from build123d import *

# Parameters (mm, degrees)
F0_W      = 711.2
F0_H      = 228.6
F0_W_2    = 685.8
F0_H_2    = 215.9
F1_DEPTH  = 381
F2_W      = 698.5
F2_H      = 136.616886
F3_DEPTH  = 190.5
F4_DEPTH  = 254
F5_W      = 203.2
F5_H      = 355.6
F6_DEPTH  = 25.4
F8_DEPTH  = 12.7
F9_W      = 698.5
F9_H      = 136.616886
F9_H_2    = 41.183114
F10_DEPTH = 381
F12_DEPTH = 25.4
F13_W     = 25.4
F13_H     = 381
F14_DEPTH = 6.35
F15_W     = 215.9
F15_H     = 120.65
F16_DEPTH = 25.4
F18_D     = 6.35
F20_D     = 12.7
F22_DEPTH = 6.35
F24_DEPTH = 6.35
F26_D     = 25.4
F28_DEPTH = 19.05
F30_D     = 12.7


with BuildPart() as f1:
    # F0 (on Top) → F1 (new body)
    with BuildSketch(Plane.XY):
        Rectangle(F0_W, F0_H)
        Rectangle(F0_W_2, F0_H_2, mode=Mode.SUBTRACT)
    extrude(amount=F1_DEPTH)

    # F2 (on face) → F3 (cut, symmetric)
    with BuildSketch(Plane.XZ.offset(114.3)):
        with Locations((0, 306.341557)):
            Rectangle(F2_W, F2_H)
    extrude(amount=F3_DEPTH, both=True, mode=Mode.SUBTRACT)

    # F2 (on face) → F4 (cut, symmetric)
    with BuildSketch(Plane.XZ.offset(114.3)):
        with BuildLine():
            Line((355.6, 0), (355.6, 190.5))
            ThreePointArc((355.6, 190.5), (153.893772, 139.874959), (0, 0))
            Line((0, 0), (355.6, 0))
        make_face()
    extrude(amount=F4_DEPTH, both=True, mode=Mode.SUBTRACT)

    # F5 (on face) → F6 (cut)
    with BuildSketch(Plane(origin=(-355.6, 0, 0), x_dir=(0, -1, 0), z_dir=(-1, 0, 0))):
        with Locations((0, 190.5)):
            Rectangle(F5_W, F5_H)
    extrude(amount=-F6_DEPTH, mode=Mode.SUBTRACT)

    # F7 (on Top) → F8 (join)
    with BuildSketch(Plane.XY):
        Polygon((-177.723765, 88.70177), (-356.087953, 88.70177), (-355.447531, -89.342214), (-177.723765, -89.342214), align=None)
    extrude(amount=F8_DEPTH)

    # F9 (on face) → F10 (cut)
    with BuildSketch(Plane.XZ.offset(114.3)):
        with Locations((0, 306.341557)):
            Rectangle(F9_W, F9_H)
        with Locations((0, 217.441557)):
            Rectangle(F9_W, F9_H_2)
    extrude(amount=-F10_DEPTH, mode=Mode.SUBTRACT)

    # F11 (on face) → F12 (cut)
    with BuildSketch(Plane.XZ.offset(114.3)):
        with BuildLine():
            Line((-177.8, 0), (0, 0))
            ThreePointArc((0, 0), (-88.9, 88.9), (-177.8, 0))
        make_face()
    extrude(amount=-F12_DEPTH, mode=Mode.SUBTRACT)

    # F13 (on face) → F14 (join)
    with BuildSketch(Plane(origin=(-355.6, 0, 0), x_dir=(0, -1, 0), z_dir=(-1, 0, 0))):
        with Locations((0, 190.5)):
            Rectangle(F13_W, F13_H)
    extrude(amount=-F14_DEPTH)

    # F15 (on face) → F16 (cut)
    with BuildSketch(Plane.YZ.offset(355.6)):
        with Locations((0, 314.325)):
            Rectangle(F15_W, F15_H)
    extrude(amount=-F16_DEPTH, mode=Mode.SUBTRACT)

    # F18 (through all)
    with Locations(Plane.YZ.offset(355.6)):
        with Locations((-86.692668, 222.25), (88.000588, 222.25)):
            Hole(F18_D / 2)

    # F20 (through all)
    with Locations(Plane(origin=(-355.6, 0, 0), x_dir=(0, -1, 0), z_dir=(-1, 0, 0))):
        with Locations((0, 296.3956), (0, 74.620992)):
            Hole(F20_D / 2)

    # F21 (on face) → F22 (join)
    with BuildSketch(Plane.XZ.offset(114.3)):
        with BuildLine():
            ThreePointArc((77.958857, 87.959228), (35.939566, 46.673864), (0, 0))
            Line((0, 0), (50.8, 0))
            Line((50.8, 0), (77.958857, 87.959228))
        make_face()
    extrude(amount=-F22_DEPTH)

    # F23 (on face) → F24 (join)
    with BuildSketch(Plane(origin=(0, 114.3, 0), x_dir=(-1, 0, 0), z_dir=(0, 1, 0))):
        with BuildLine():
            ThreePointArc((0, 0), (-35.80659, 46.523758), (-77.65419, 87.69839))
            Line((-77.65419, 87.69839), (-50.599013, 0))
            Line((-50.599013, 0), (0, 0))
        make_face()
    extrude(amount=-F24_DEPTH)

    # F26 (through all)
    with Locations(Plane(origin=(0, 114.3, 0), x_dir=(-1, 0, 0), z_dir=(0, 1, 0))):
        with Locations((-25.399767, 34.288563)):
            Hole(F26_D / 2)

    # F27 (on face) → F28 (join)
    with BuildSketch(Plane(origin=(0, 0, 0), x_dir=(1, 0, 0), z_dir=(0, 0, -1))):
        Polygon((-355.837416, -19.05), (-355.700371, 19.049877), (-622.535691, 20.00968), (-622.535691, -18.090689), align=None)
    extrude(amount=-F28_DEPTH)

    # F30 (through all)
    with Locations(Plane.XY.offset(19.05)):
        with Locations((-555.843129, -0.959495), (-422.458004, -0.959495)):
            Hole(F30_D / 2)


solid = f1.part
Here's how the part is built. I have some questions about the finished solid (model axes, mm). A direction names the side the tool comes from. Coordinates: 2 decimals unless noted, no trailing zeros. Order: outer loops, then holes, each group sorted by start corner. A loop starts at its lowest first (then second) coordinate and runs counter-clockwise, first axis right, second up. Notation, with made-up numbers: M -7,56.5 L 16,56.5 A20 cw 16,73.5 Z; hole C -2,2.25 d4. An arc over 180 degrees is marked long. Answer as CSV lines item,"result". Start each with the question number.
1. On a 3-axis mill with a long thin cutter (end or side, diameter ignored), from which of +Z, -Z, +X, -X, +Y, -Y can I reach the whole of each face in a straight line? I mean faces 1 (the flat face through (-107, 111, 381)), 2 (the flat face through (-2, -111, 196.85)), 3 (the cylindrical face through (-86.95, -111.17, 88.88)), 4 (the flat face through (-349.25, -9, 248)). Say none if no direction works.
2. I want a section at B-B, the plane x = -88.9. Write out the boundary of the cut face in (y, z).
3. I want a section at A-A, the plane y = -74. Write out the boundary of the cut face in (x, z).
4. For pin 1 (2 mm diameter, centred on x = -302.5, y = 65, fed in from +Z); pin 2 (19.5 mm diameter, centred on x = -518.5, y = -8, fed in from +Z); pin 3 (6 mm diameter, centred on y = 0, z = 241.5, fed in from -X); pin 4 (10 mm diameter, centred on x = -346.5, z = 244.5, fed in from -Y), each with a flat end and sliding along its axis, tell me the tip position at first contact or that it passes through.
5. We'd pull the mould along X, two halves only. Please class faces 5 (the cylindrical face through (350.7, -0.53, 190.47)), 6 (the flat face through (-74, 114.3, 109)), 7 (the cylindrical face through (22.6, 111.1, 21.9)): released by +X, released by -X, zero draft, split by the parting line, or undercut.
6. I want a section at D-D, the plane x = 192. Write out the boundary of the cut face in (y, z).
7. I need wall thicknesses on line 1 (Y direction, x = 354, z = 222.25); line 2 (Y direction, x = -185, z = 191). Which ranges of each line are inside material? Lowest first, please. Write a range as [from, to].
8. I want a section at C-C, the plane y = 53.5. Write out the boundary of the cut face in (x, z), and give its area (3 significant figures).
Recorded:
1,face 1,"+Z, +X, -X, +Y, -Y"
1,face 2,"+Y, -Y"
1,face 3,"-Z, -Y"
1,face 4,"none"
2,outline,"M -114.3,88.9 L -107.95,88.9 L -107.95,196.85 L -114.3,196.85 Z; M -114.3,374.65 L -107.95,374.65 L -107.95,381 L -114.3,381 Z; M 107.95,0 L 114.3,0 L 114.3,196.85 L 107.95,196.85 Z; M 107.95,374.65 L 114.3,374.65 L 114.3,381 L 107.95,381 Z"
3,outline,"M -355.6,0 L -177.72,0 L -177.72,12.7 L -355.6,12.7 Z; M -355.6,368.3 L -349.25,368.3 L -349.25,374.65 L -342.9,374.65 L -342.9,381 L -355.6,381 Z; M 342.9,190.31 A427.14 cw 355.6,190.5 L 355.6,254 L 349.25,254 L 349.25,196.85 L 342.9,196.85 Z; M 342.9,374.65 L 355.6,374.65 L 355.6,381 L 342.9,381 Z"
4,pin 1,"stops at z = 12.7"
4,pin 2,"stops at z = 19.05"
4,pin 3,"stops at x = -355.6"
4,pin 4,"stops at y = -114.3"
5,face 5,"released by +X"
5,face 6,"zero draft"
5,face 7,"undercut"
6,outline,"M -114.3,157.93 L -107.95,157.93 L -107.95,196.85 L -114.3,196.85 Z; M -114.3,374.65 L -107.95,374.65 L -107.95,381 L -114.3,381 Z; M 107.95,157.93 L 114.3,157.93 L 114.3,196.85 L 107.95,196.85 Z; M 107.95,374.65 L 114.3,374.65 L 114.3,381 L 107.95,381 Z"
7,line 1,"y = [-114.3, -89.87], [-83.52, 84.83], [91.18, 114.3]"
7,line 2,"y = [-114.3, -107.95], [107.95, 114.3]"
8,outline,"M -355.96,0 L -177.72,0 L -177.72,12.7 L -355.96,12.7 Z; M -355.6,368.3 L -349.25,368.3 L -349.25,374.65 L -342.9,374.65 L -342.9,381 L -355.6,381 Z; M 342.9,190.31 A427.14 cw 355.6,190.5 L 355.6,254 L 349.25,254 L 349.25,196.85 L 342.9,196.85 Z; M 342.9,374.65 L 355.6,374.65 L 355.6,381 L 342.9,381 Z"
8,area,"2,910 mm2"
